Read the model definition and answer for the solid it produces. Units are mm, in the model's axes. Round coordinates to 2 decimals unless told otherwise and drop trailing zeros. Loops run counter-clockwise (first coordinate to the right, second up) from the corner with the lowest first, then second, coordinate; pieces in that order, holes last. Notation, with made-up numbers: (5.25, 31) - (64.25, 31) arc R22 cw to (64.25, 47) - close; hole circle Ø8 at (57, -22.5). An arc over 180 degrees is marked (long way). Use CSV: the item, a comma, the result in double quotes. Start each with the question number.
1. Find section A-A (y = 0). Give the vertices of the cut face in (x, z), and give its area (3 significant figures).
2. Find section C-C (z = 0). Give the vertices of the cut face in (x, y).
3. Given pin 1 Ø3.5 at (x, y) = (0, 0) entering from +Z, flat-ended and moving along its own axis, determine where the tip first touches the part or whether it passes through.
4. Consider line 1 along Y through (x, z) = (0, -0.05); line 2 along Y through (x, z) = (-1, 0.3). Determine where each line is inside the solid, lowest interval first.
5. Determine the mould class of faces 1 (the cylindrical face through (-2.15, 0.09, 0)), 2 (the cylindrical face through (-0.59, 4.46, 0)), 3 (the flat face through (2, -2, 0.4)) for opening direction Y: +Y half, -Y half, draft (parallel to the pull), parting line (faces both ways), or undercut.
from build123d import *

# Parameters (mm, degrees)
BOSS_EXTRUDE1_START = 0.4
SKETCH3_R           = 4.5
SKETCH3_R_2         = 2.15
BOSS_EXTRUDE1_DEPTH = 0.8
FILLET1_R           = 0.06


with BuildPart() as part:
    # Sketch3 → Boss-Extrude1 (new body)
    with BuildSketch(Plane.XY.offset(BOSS_EXTRUDE1_START)):
        Circle(SKETCH3_R)
        Circle(SKETCH3_R_2, mode=Mode.SUBTRACT)
    extrude(amount=-BOSS_EXTRUDE1_DEPTH)

    # Fillet1
    fillet1_edges = [part.edges().sort_by_distance(p)[0] for p in [
        (-4.5, 0, 0.4),
        (-4.5, 0, -0.4),
        (-2.15, 0, -0.4),
        (-2.15, 0, 0.4),
    ]]
    fillet(fillet1_edges, radius=FILLET1_R)


solid = part.part
Filled sheet:
1,outline,"(-4.5, -0.34) arc R0.06 ccw to (-4.44, -0.4) - (-2.21, -0.4) arc R0.06 ccw to (-2.15, -0.34) - (-2.15, 0.34) arc R0.06 ccw to (-2.21, 0.4) - (-4.44, 0.4) arc R0.06 ccw to (-4.5, 0.34) - close; (2.15, -0.34) arc R0.06 ccw to (2.21, -0.4) - (4.44, -0.4) arc R0.06 ccw to (4.5, -0.34) - (4.5, 0.34) arc R0.06 ccw to (4.44, 0.4) - (2.21, 0.4) arc R0.06 ccw to (2.15, 0.34) - close"
1,area,"3.75 mm²"
2,outline,"circle Ø9 at (0, 0); hole circle Ø4.3 at (0, 0)"
3,pin 1,"passes through"
4,line 1,"y = -4.5 to -2.15, 2.15 to 4.5"
4,line 2,"y = -4.39 to -1.9, 1.9 to 4.39"
5,face 1,"undercut"
5,face 2,"parting line"
5,face 3,"draft"
